Here's how the part is built. I have some questions about the finished solid (model axes, mm). A direction names the side the tool comes from. Round coordinates to 2 decimals unless told otherwise and drop trailing zeros. Write each loop counter-clockwise with the first axis right and the second up, starting at its lowest first coordinate (ties: lowest second). Pieces come first, ordered by that corner, then holes. Notation, with made-up numbers: (66.25, -2) -> (89.25, -2) arc R25 cw to (89.25, 36) -> close; hole circle Ø3 at (39, 88.25). An arc over 180 degrees is marked (long way). Put each result on its own line as item: value. Start each with the question number.
1) I want a section at C-C, the plane y = 149.5. List the corners of the cut face in (x, z) for me, then the cut area to 3 significant figures.
2) We'd pull the mould along X, two halves only. Please class faces 1 (the cylindrical face through (17.003, 109.145, -32.978)), 2 (the flat face through (-10.7, 131.4, -50)), 3 (the cylindrical face through (-20.387, 117.092, -32.477)): released by +X, released by -X, zero draft, split by the parting line, or undercut.
3) I want a section at D-D, the plane x = -15. Give the number of separate pieces and of enclosed holes in the cut face, then the cut area to 3 significant figures.
4) Which directions (+Z, -Z, +X, -X, +Y, -Y) give clear straight access to the entire face, cutting with the end or side of a thin tool? Please do faces 4 (the cylindrical face through (-0.848, 243.865, -0.155)), 5 (the flat face through (16, 0, -11)), 6 (the flat face through (-30, 226, -9.532)), 7 (the flat face through (-7.6, 216.389, -23.2)), 8 (the flat face through (0, 242, 11.05)).
5) I want a section at A-A, the plane z = 32. List the corners of the cut face in (x, y) for me.
6) I want a section at B-B, the plane x = -56. List the corners of the cut face in (y, z) for me.
7) If I drill on line 1 along Y through (x, z) = (0, 39); line 2 along Y through (x, z) = (0, -20.5); line 3 along Y through (x, z) = (1.5, -30.5), over which ranges is the centre line in solid material (lowest first)? Write a range as [from, to].
8) Will these pins go through, and if not, where does the flat tip stop? P1, Ø12, axis at y = 81.5, z = 23, coming from the -X side; P2, Ø8, axis at x = -33, z = 24, coming from the +Y side; P3, Ø1.5, axis at x = -22, y = 216, coming from the -Z side.
from build123d import *

# Parameters (mm, degrees)
SKETCH7_R           = 21.1979112
BOSS_EXTRUDE1_DEPTH = 180.647627
SKETCH12_R          = 20.406966807
BOSS_EXTRUDE6_DEPTH = 50
SHELL1_START        = -50
SHELL1_OUTLINE_R    = 18.406966807
SHELL1_DEPTH        = 100
SHELL1_2_OUTLINE_R  = 19.1979112
SHELL1_2_DEPTH      = 178.6476265
SKETCH8_R           = 47.3804642
BOSS_EXTRUDE2_DEPTH = 4.431169
SKETCH9_R           = 24.21431875
BOSS_EXTRUDE3_DEPTH = 31.309755
SKETCH10_R          = 25.98338315
BOSS_EXTRUDE4_DEPTH = 19.395214
CHAMFER1_SIZE       = 4
SKETCH11_R          = 3.909700179
BOSS_EXTRUDE5_DEPTH = 11.05
SKETCH13_W          = 19.064805676
SKETCH13_H          = 16.075701836
BOSS_EXTRUDE7_DEPTH = 52
SKETCH14_R          = 17.318879346
SKETCH14_R_2        = 11.636848892
SKETCH14_R_3        = 5.411731441
CUT_EXTRUDE1_DEPTH  = 26
SKETCH14_5_R        = 17.318879346
SKETCH14_5_R_2      = 5.411731441
BOSS_EXTRUDE9_DEPTH = 6


with BuildPart() as part:
    # Sketch7 → Boss-Extrude1 (new body)
    with BuildSketch(Plane(origin=(0, 0, 0), x_dir=(1, 0, 0), z_dir=(0, 1, 0))):
        with Locations(Location((0, 0, 0), (0, 0, 270))):
            Circle(SKETCH7_R)
    extrude(amount=BOSS_EXTRUDE1_DEPTH)

    # Sketch12 → Boss-Extrude6 (add, symmetric)
    with BuildSketch(Plane.XY):
        with Locations((0, 116.195122616)):
            Circle(SKETCH12_R)
    extrude(amount=BOSS_EXTRUDE6_DEPTH, both=True)

    # Shell1: read off the stored shape, not the designer's step
    # Shell1 outline → Shell1 (cut)
    with BuildSketch(Plane.XY.offset(SHELL1_START)):
        with Locations((0, 116.195122616)):
            Circle(SHELL1_OUTLINE_R)
    extrude(amount=SHELL1_DEPTH, mode=Mode.SUBTRACT)

    # Shell1 2 outline → Shell1 2 (cut)
    with BuildSketch(Plane(origin=(0, 0, 0), x_dir=(1, 0, 0), z_dir=(0, 1, 0))):
        Circle(SHELL1_2_OUTLINE_R)
    extrude(amount=SHELL1_2_DEPTH, mode=Mode.SUBTRACT)

    # Sketch8 → Boss-Extrude2 (add)
    with BuildSketch(Plane(origin=(0, 180.6476265, 0), x_dir=(1, 0, 0), z_dir=(0, 1, 0))):
        with Locations(Location((0, 0, 0), (0, 0, 270))):
            Circle(SKETCH8_R)
    extrude(amount=BOSS_EXTRUDE2_DEPTH)

    # Sketch9 → Boss-Extrude3 (add)
    with BuildSketch(Plane(origin=(0, 185.0787951, 0), x_dir=(1, 0, 0), z_dir=(0, 1, 0))):
        with Locations(Location((0, 0, 0), (0, 0, 270))):
            Circle(SKETCH9_R)
    extrude(amount=BOSS_EXTRUDE3_DEPTH)

    # Sketch10 → Boss-Extrude4 (add)
    with BuildSketch(Plane(origin=(0, 216.3885498, 0), x_dir=(1, 0, 0), z_dir=(0, 1, 0))):
        with Locations(Location((0, 0, 0), (0, 0, 270))):
            Circle(SKETCH10_R)
    extrude(amount=BOSS_EXTRUDE4_DEPTH)

    # Chamfer1
    chamfer1_edges = [part.edges().sort_by_distance(p)[0] for p in [
        (0, 185.0787951, -24.21431875),
    ]]
    chamfer(chamfer1_edges, length=CHAMFER1_SIZE)

    # Sketch11 → Boss-Extrude5 (add, symmetric)
    with BuildSketch(Plane.XY):
        with BuildLine():
            Line((-18.74694623, 235.7837635), (18.74694623, 235.7837635))
            add(Edge.make_bspline(
                [(18.74694623, 235.7837635), (13.888692834, 253.685965272), (8.293919463, 257.014643256), (0, 257.491213049)],
                knots=[0, 0, 0, 0, 0.516374354, 0.516374354, 0.516374354, 0.516374354], degree=3))
            add(Edge.make_bspline(
                [(-18.74694623, 235.7837635), (-13.888692834, 253.685965272), (-8.293919463, 257.014643256), (0, 257.491213049)],
                knots=[0, 0, 0, 0, 0.516374354, 0.516374354, 0.516374354, 0.516374354], degree=3))
        make_face()
        with Locations((0, 247.681579845)):
            Circle(SKETCH11_R, mode=Mode.SUBTRACT)
    extrude(amount=BOSS_EXTRUDE5_DEPTH, both=True)

    # Sketch13 → Boss-Extrude7 (add)
    with BuildSketch(Plane(origin=(0, 0, 0), x_dir=(0, 0, -1), z_dir=(1, 0, 0))):
        with Locations((0, 226.08615665)):
            Rectangle(SKETCH13_W, SKETCH13_H)
    extrude(amount=-BOSS_EXTRUDE7_DEPTH)

    # Sketch14 → Cut-Extrude1 (cut, symmetric)
    # profile 1 of 2: a face of its own
    with BuildSketch(Plane.XY):
        with Locations((-53.889606886, 223.55520268)):
            Circle(SKETCH14_R)
        with Locations((-53.889606886, 223.55520268)):
            Circle(SKETCH14_R_2, mode=Mode.SUBTRACT)
    # profile 2 of 2: a face of its own
    with BuildSketch(Plane.XY):
        with Locations((-53.889606886, 223.55520268)):
            Circle(SKETCH14_R_3)
    extrude(amount=CUT_EXTRUDE1_DEPTH, both=True, mode=Mode.SUBTRACT)


with BuildPart() as cut_extrude1_kept_piece:
    # of the separate pieces the step leaves, the one the design keeps (cut_extrude1_pieces_kept)
    add(part.part.solids().sort_by_distance((0, 189.0787955, 24.21431875))[0])

    # Sketch14<5> → Boss-Extrude9 (add, symmetric)
    with BuildSketch(Plane.XY):
        with Locations((-53.889606886, 223.55520268)):
            Circle(SKETCH14_5_R)
        with Locations((-53.889606886, 223.55520268)):
            Circle(SKETCH14_5_R_2, mode=Mode.SUBTRACT)
    extrude(amount=BOSS_EXTRUDE9_DEPTH, both=True)


solid = cut_extrude1_kept_piece.part
Findings:
1. outline: circle Ø42.4 at (0, 0); hole circle Ø38.4 at (0, 0)
1. area: 254 mm2
2. face 1: undercut
2. face 2: zero draft
2. face 3: split by the parting line
3. separate pieces: 3
3. enclosed holes: 0
3. area: 4,120 mm2
4. face 4: +Z, -Z
4. face 5: +Z, -Z, +X, -X, -Y
4. face 6: -Z, -X, +Y
4. face 7: none
4. face 8: +Z, +X, -X, +Y
5. outline: (-34.94, 180.65) -> (34.94, 180.65) -> (34.94, 185.08) -> (-34.94, 185.08) -> close; circle Ø40.81 at (0, 116.2); hole circle Ø36.81 at (0, 116.2)
6. outline: (206.37, -6) -> (218.57, -6) -> (218.57, 6) -> (206.37, 6) -> close; (228.54, -6) -> (240.75, -6) -> (240.75, 6) -> (228.54, 6) -> close
7. line 1: y = [95.79, 97.79], [134.6, 136.6], [180.65, 185.08]
7. line 2: y = [0, 97.79], [134.6, 235.78]
7. line 3: y = [95.84, 97.85], [134.54, 136.55], [180.65, 185.08]
8. P1: stops at x = -12.66
8. P2: stops at y = 185.08
8. P3: stops at z = -14.8
